Check sheet for the modelled part. Datum: model origin and axes. Units: mm. A direction names the side the tool comes from. Give positions to 0.01 mm unless a question says otherwise; leave off trailing zeros. Write each loop counter-clockwise with the first axis right and the second up, starting at its lowest first coordinate (ties: lowest second). Pieces come first, ordered by that corner, then holes. Notation, with made-up numbers: (-18, 37.5) -> (36, 37.5) arc R26 ccw to (36, 72.5) -> close; hole circle Ø2 at (22, 67.25). An arc over 180 degrees is marked (long way). Return JSON: item names as keys, results as strings.
from build123d import *

# Parameters (mm, degrees)
BOSS_EXTRUDE4_DEPTH = 0.2
BOSS_EXTRUDE5_DEPTH = 0.35
BOSS_EXTRUDE6_DEPTH = 0.5
SKETCH5_W           = 21.158330311
SKETCH5_H           = 11.75153324
BOSS_EXTRUDE7_DEPTH = 1
SKETCH8_W           = 25.80987528
SKETCH8_H           = 15.757102731
SKETCH8_W_2         = 21.158330311
SKETCH8_H_2         = 11.75153324
BOSS_EXTRUDE8_DEPTH = 3.5


with BuildPart() as part:
    # Sketch1 → Boss-Extrude4 (new body)
    with BuildSketch(Plane.XY):
        with BuildLine():
            Line((-4.8, 0.09272626), (-5.796194698, 0.179882003))
            ThreePointArc((-5.796194698, 0.179882003), (-5.983350441, -0.00727374), (-5.796194698, -0.194429483))
            Line((-5.796194698, -0.194429483), (-4.8, -0.10727374))
            Line((-4.8, -0.10727374), (-2.8, -0.10727374))
            Line((-2.8, -0.10727374), (-2.8, 0.09272626))
            Line((-2.8, 0.09272626), (-4.8, 0.09272626))
        make_face()
    extrude(amount=BOSS_EXTRUDE4_DEPTH)

    # Sketch1<7> → Boss-Extrude5 (add)
    with BuildSketch(Plane.XY):
        with BuildLine():
            Line((-2.8, 0.29272626), (-2.8, 0.09272626))
            Line((-2.8, 0.09272626), (-2.8, -0.10727374))
            Line((-2.8, -0.10727374), (-2.8, -0.30727374))
            Line((-2.8, -0.30727374), (-3.4, -0.30727374))
            Line((-3.4, -0.30727374), (-4.999165526, -1.623297206))
            ThreePointArc((-4.999165526, -1.623297206), (-5.02151566, -1.853410903), (-4.791401964, -1.875761037))
            Line((-4.791401964, -1.875761037), (-3.25, -0.60727374))
            Line((-3.25, -0.60727374), (-2.5, -0.60727374))
            Line((-2.5, -0.60727374), (-2.5, -0.10727374))
            Line((-2.5, -0.10727374), (0, -0.10727374))
            Line((0, -0.10727374), (0, 0.09272626))
            Line((0, 0.09272626), (-2.5, 0.09272626))
            Line((-2.5, 0.09272626), (-2.5, 0.59272626))
            Line((-2.5, 0.59272626), (-3.25, 0.59272626))
            Line((-3.25, 0.59272626), (-4.791401964, 1.861213558))
            ThreePointArc((-4.791401964, 1.861213558), (-5.02151566, 1.838863423), (-4.999165526, 1.608749727))
            Line((-4.999165526, 1.608749727), (-3.4, 0.29272626))
            Line((-3.4, 0.29272626), (-2.8, 0.29272626))
        make_face()
    extrude(amount=BOSS_EXTRUDE5_DEPTH)

    # Sketch1<8> → Boss-Extrude6 (add)
    with BuildSketch(Plane.XY):
        with BuildLine():
            Line((0, 0.29272626), (0, -0.30727374))
            Line((0, -0.30727374), (-0.6, -0.30727374))
            Line((-0.6, -0.30727374), (-2.199165526, -1.623297206))
            ThreePointArc((-2.199165526, -1.623297206), (-2.22151566, -1.853410903), (-1.991401964, -1.875761037))
            Line((-1.991401964, -1.875761037), (-0.45, -0.60727374))
            Line((-0.45, -0.60727374), (0.3, -0.60727374))
            Line((0.3, -0.60727374), (0.3, -0.10727374))
            Line((0.3, -0.10727374), (2, -0.10727374))
            Line((2, -0.10727374), (2, 2.090619677))
            Line((2, 2.090619677), (2.2, 2.090619677))
            Line((2.2, 2.090619677), (2.2, -2.409380323))
            Line((2.2, -2.409380323), (2.8, -2.409380323))
            Line((2.8, -2.409380323), (2.8, 2.090619677))
            Line((2.8, 2.090619677), (3, 2.090619677))
            Line((3, 2.090619677), (3, -2.409380323))
            Line((3, -2.409380323), (3.6, -2.409380323))
            Line((3.6, -2.409380323), (3.6, 2.090619677))
            Line((3.6, 2.090619677), (3.8, 2.090619677))
            Line((3.8, 2.090619677), (3.8, -2.409380323))
            Line((3.8, -2.409380323), (4.4, -2.409380323))
            Line((4.4, -2.409380323), (4.4, 2.090619677))
            Line((4.4, 2.090619677), (4.6, 2.090619677))
            Line((4.6, 2.090619677), (4.6, -2.409380323))
            Line((4.6, -2.409380323), (5.2, -2.409380323))
            Line((5.2, -2.409380323), (5.2, 2.090619677))
            Line((5.2, 2.090619677), (5.4, 2.090619677))
            Line((5.4, 2.090619677), (5.4, -2.409380323))
            Line((5.4, -2.409380323), (6, -2.409380323))
            Line((6, -2.409380323), (6, 2.090619677))
            Line((6, 2.090619677), (6.2, 2.090619677))
            Line((6.2, 2.090619677), (6.2, -2.409380323))
            Line((6.2, -2.409380323), (6.8, -2.409380323))
            Line((6.8, -2.409380323), (6.8, 2.090619677))
            Line((6.8, 2.090619677), (7, 2.090619677))
            Line((7, 2.090619677), (7, -2.409380323))
            Line((7, -2.409380323), (7.6, -2.409380323))
            Line((7.6, -2.409380323), (7.6, -0.159380323))
            Line((7.6, -0.159380323), (9.6, -0.159380323))
            Line((9.6, -0.159380323), (10.098097349, -0.202958194))
            ThreePointArc((10.098097349, -0.202958194), (10.242728512, -0.058327031), (10.098097349, 0.086304132))
            Line((10.098097349, 0.086304132), (9.6, 0.04272626))
            Line((9.6, 0.04272626), (7.4, 0.04272626))
            Line((7.4, 0.04272626), (7.4, -2.20727374))
            Line((7.4, -2.20727374), (7.2, -2.20727374))
            Line((7.2, -2.20727374), (7.2, 2.29272626))
            Line((7.2, 2.29272626), (6.6, 2.29272626))
            Line((6.6, 2.29272626), (6.6, -2.20727374))
            Line((6.6, -2.20727374), (6.4, -2.20727374))
            Line((6.4, -2.20727374), (6.4, 2.29272626))
            Line((6.4, 2.29272626), (5.8, 2.29272626))
            Line((5.8, 2.29272626), (5.8, -2.20727374))
            Line((5.8, -2.20727374), (5.6, -2.20727374))
            Line((5.6, -2.20727374), (5.6, 2.29272626))
            Line((5.6, 2.29272626), (5, 2.29272626))
            Line((5, 2.29272626), (5, -2.20727374))
            Line((5, -2.20727374), (4.8, -2.20727374))
            Line((4.8, -2.20727374), (4.8, 2.29272626))
            Line((4.8, 2.29272626), (4.2, 2.29272626))
            Line((4.2, 2.29272626), (4.2, -2.20727374))
            Line((4.2, -2.20727374), (4, -2.20727374))
            Line((4, -2.20727374), (4, 2.29272626))
            Line((4, 2.29272626), (3.4, 2.29272626))
            Line((3.4, 2.29272626), (3.4, -2.20727374))
            Line((3.4, -2.20727374), (3.2, -2.20727374))
            Line((3.2, -2.20727374), (3.2, 2.29272626))
            Line((3.2, 2.29272626), (2.6, 2.29272626))
            Line((2.6, 2.29272626), (2.6, -2.20727374))
            Line((2.6, -2.20727374), (2.4, -2.20727374))
            Line((2.4, -2.20727374), (2.4, 2.29272626))
            Line((2.4, 2.29272626), (1.8, 2.29272626))
            Line((1.8, 2.29272626), (1.8, 0.09272626))
            Line((1.8, 0.09272626), (0.3, 0.09272626))
            Line((0.3, 0.09272626), (0.3, 0.59272626))
            Line((0.3, 0.59272626), (-0.45, 0.59272626))
            Line((-0.45, 0.59272626), (-1.991401964, 1.861213558))
            ThreePointArc((-1.991401964, 1.861213558), (-2.22151566, 1.838863423), (-2.199165526, 1.608749727))
            Line((-2.199165526, 1.608749727), (-0.6, 0.29272626))
            Line((-0.6, 0.29272626), (0, 0.29272626))
        make_face()
    extrude(amount=BOSS_EXTRUDE6_DEPTH)

    # Sketch5 → Boss-Extrude7 (add)
    with BuildSketch(Plane(origin=(0, 0, 0), x_dir=(-1, 0, 0), z_dir=(0, 0, -1))):
        with Locations((-2.065173388, -0.096435412)):
            Rectangle(SKETCH5_W, SKETCH5_H)
    extrude(amount=BOSS_EXTRUDE7_DEPTH)

    # Sketch8 → Boss-Extrude8 (add)
    with BuildSketch(Plane(origin=(0, 0, -1), x_dir=(-1, 0, 0), z_dir=(0, 0, -1))):
        with Locations((-2.067728751, -0.024369167)):
            Rectangle(SKETCH8_W, SKETCH8_H)
        with Locations((-2.065173388, -0.096435412)):
            Rectangle(SKETCH8_W_2, SKETCH8_H_2, mode=Mode.SUBTRACT)
    extrude(amount=-BOSS_EXTRUDE8_DEPTH)


solid = part.part
(1) Cross-section at A-A on z = 2.15. Enter the section's corners in (x, y), then the cut area to 3 significant figures.
Reply:
{"outline": "(-10.84, -7.9) -> (14.97, -7.9) -> (14.97, 7.85) -> (-10.84, 7.85) -> close; hole (-8.51, -5.97) -> (12.64, -5.97) -> (12.64, 5.78) -> (-8.51, 5.78) -> close", "area": "158 mm^2"}
(2) Cross-section at C-C on y = -3.75. Enter the section's corners in (x, z).
Reply:
{"outline": "(-10.84, -1) -> (14.97, -1) -> (14.97, 2.5) -> (12.64, 2.5) -> (12.64, 0) -> (-8.51, 0) -> (-8.51, 2.5) -> (-10.84, 2.5) -> close"}
(3) Thickness scan on L1, parallel to Y at x = -1, z = 0.7; L2, parallel to X at y = -3.5, z = 0.2; L3, parallel to Z at x = -5.75, y = 2.75. Record the ranges inside material, lowest first.
Reply:
{"L1": "-7.9 to -5.97, 5.78 to 7.85", "L2": "-10.84 to -8.51, 12.64 to 14.97", "L3": "-1 to 0"}
(4) Cross-section at D-D on x = -5.5. Enter the section's corners in (y, z).
Reply:
{"outline": "(-7.9, -1) -> (7.85, -1) -> (7.85, 2.5) -> (5.78, 2.5) -> (5.78, 0) -> (0.15, 0) -> (0.15, 0.2) -> (-0.17, 0.2) -> (-0.17, 0) -> (-5.97, 0) -> (-5.97, 2.5) -> (-7.9, 2.5) -> close"}
(5) Release check for a two-part mould opening along Y. For faces 3 (the flat face through (2, -7, 2.5)), 4 (the flat face through (-4.03, -1.25, 0.17)), 5 (the flat face through (2, 7.854, 1)) record: pulls with the +Y half, pulls with the -Y half, needs draft (parallel to the pull), parting line crosses it, or undercut.
Reply:
{"face 3": "needs draft", "face 4": "undercut", "face 5": "pulls with the +Y half"}
(6) Cross-section at B-B on x = 10.75. Enter the section's corners in (y, z), then the cut area to 3 significant figures.
Reply:
{"outline": "(-7.9, -1) -> (7.85, -1) -> (7.85, 2.5) -> (5.78, 2.5) -> (5.78, 0) -> (-5.97, 0) -> (-5.97, 2.5) -> (-7.9, 2.5) -> close", "area": "25.8 mm^2"}
(7) Set-up check for faces 1 (the flat face through (-4.21, 0.96, 0.17)), 2 (the flat face through (-10.837, 0, 1)): record each of +Z, -Z, +X, -X, +Y, -Y from which the full face is reachable in a straight line by a thin tool's end or side.
Reply:
{"face 1": "+Z", "face 2": "+Z, -Z, -X, +Y, -Y"}
